For this review, take the finished solid that the model builds, in its own axes (mm). A direction names the side the tool comes from. Round coordinates to 2 decimals unless told otherwise and drop trailing zeros. Write each loop counter-clockwise with the first axis right and the second up, starting at its lowest first coordinate (ties: lowest second). Pieces come first, ordered by that corner, then holes. Notation, with made-up numbers: M 39,9.5 L 82,9.5 A14 ccw 82,22.5 Z; hole C -14,-6.75 d10. An arc over 180 degrees is marked long. Use one line per item in the form item = value. Start each with the question number.
Item 1: Add section B-B (z = 16). State the section outline as (x, y) points (3 decimals).
Item 2: For P1, Ø5, axis at y = 4.5, z = 2, coming from the +X side; P2, Ø2.5, axis at y = 10.91, z = 29.1, coming from the +X side; P3, Ø11.5, axis at y = 20, z = 20, coming from the -X side; P4, Ø3, axis at x = 6.5, z = 16, coming from the +Y side, all flat-tipped, find the tip position at first contact; note any pin that passes through.
Item 3: For line 1 (Z direction, x = 2.5, y = 36.83) (1 decimal); line 2 (Z direction, x = 6, y = 36.5); line 3 (X direction, y = 4, z = 7), list the stretches that pass through material, from the lowest coordinate up. Write a range as [from, to].
Item 4: Add section A-A (y = 19). State the section outline as (x, z) points (3 decimals).
Item 5: Draft analysis for pull direction Y (two halves, no side actions). For faces 1 (the cylindrical face through (3.256, 3.128, 4.253)), 2 (the cylindrical face through (1.25, 28.09, 11.04)), 3 (the flat face through (1, 40.005, 12)), 4 (the flat face through (1, 20, 0)), state which applies: released by +Y, released by -Y, zero draft, split by the parting line, or undercut.
Item 6: Add section C-C (x = 3.25). Count the separate pieces of the cut face and the enclosed holes in it, and give its area (3 significant figures).
Item 7: For faces 5 (the flat face through (1, 40.005, 36)), 6 (the flat face through (6.985, 20, 30)), 7 (the cylindrical face through (6.484, 16.855, 10.009)), list the 3-axis set-ups (+Z, -Z, +X, -X, +Y, -Y) from which the entire face can be reached by the end or side of a thin tool; tool diameter is ignored.
Item 8: Add section D-D (z = 11). State the section outline as (x, y) points (3 decimals).
Autodesk Inventor part; units mm, degrees
ref_plane "YZ Plane" through (0, 0, 0) normal (1, 0, 0) x (0, 1, 0)
ref_plane "XZ Plane" through (0, 0, 0) normal (0, 1, 0) x (-1, 0, 0)
ref_plane "XY Plane" through (0, 0, 0) normal (0, 0, 1) x (1, 0, 0)
sketch "Sketch1" plane through (0, 0, 0) normal (1, 0, 0) x (0, 1, 0)
  line L0 (0, 0) -> (40.005, 0)
  line L1 (40.005, 0) -> (40.005, 40.005)
  line L2 (40.005, 40.005) -> (0, 40.005)
  line L3 (0, 40.005) -> (0, 0)
  dimension "d0" = 40.005
  dimension "d1" = 40.005
extrude "Extrusion1" add sketch "Sketch1" along normal blind 2.54
fillet "Fillet1" radius 3.175 4 edges at (1.27, 40.005, 40.005) (1.27, 0, 40.005) (1.27, 0, 0) (1.27, 40.005, 0)
sketch "Sketch2" plane through (2.54, 0, 0) normal (1, 0, 0) x (0, 0, -1)
  arc A0 (0, 36.83) -> (-3.175, 40.005) centre (-3.175, 36.83) ccw
  arc A1 (-36.83, 40.005) -> (-40.005, 36.83) centre (-36.83, 36.83) ccw
  arc A2 (-40.005, 3.175) -> (-36.83, 0) centre (-36.83, 3.175) ccw
  arc A3 (-3.175, 0) -> (0, 3.175) centre (-3.175, 3.175) ccw
  circle A4 centre (-36.83, 3.175) radius 3.175
  circle A5 centre (-36.83, 36.83) radius 3.175
  circle A6 centre (-3.175, 36.83) radius 3.175
  circle A7 centre (-3.175, 3.175) radius 3.175
  point P0 (0, 0)
extrude "Extrusion2" add sketch "Sketch2" along normal blind 4.064
sketch "Sketch3" plane through (6.604, 3.175, 36.83) normal (1, 0, 0) x (0, 0, -1)
  circle A0 centre (0, 0) radius 3.175
  circle A1 centre (0, 33.655) radius 3.175
  circle A2 centre (33.655, 33.655) radius 3.175
  circle A3 centre (33.655, 0) radius 3.175
  point P0 (36.83, -3.175)
hole "Hole1" at (6.604, 36.83, 36.83) at (6.604, 36.83, 3.175) at (6.604, 3.175, 3.175) at (6.604, 3.175, 36.83) direction (-1, 0, 0) diameter 2.159 end through all
sketch "Sketch4" plane through (2.54, 0, 0) normal (1, 0, 0) x (0, 0, -1)
  arc A0 (-3.175, 40.005) -> (0, 36.83) centre (-3.175, 36.83) ccw
  arc A1 (-36.83, 0) -> (-40.005, 3.175) centre (-36.83, 3.175) ccw
  line L0 (-10.9093, 10.9093) -> (-29.0957, 10.9093)
  line L1 (-29.0957, 10.9093) -> (-29.0957, 29.0957)
  line L2 (-29.0957, 29.0957) -> (-10.9093, 29.0957)
  line L3 (-10.9093, 29.0957) -> (-10.9093, 10.9093)
  line L4 (-36.83, 3.175) -> (-3.175, 36.83) construction
  line L5 (-10.9093, 10.9093) -> (-29.0957, 29.0957) construction
  point P0 (0, 0)
  point P1 (-20.0025, 20.0025)
  dimension "d14" = 18.1864
hole "Hole2" at (2.54, 10.9093, 29.0957) at (2.54, 29.0957, 29.0957) at (2.54, 10.9093, 10.9093) at (2.54, 29.0957, 10.9093) direction (-1, 0, 0) diameter 2.032 end through all
sketch "Sketch5" plane through (2.54, 0, 0) normal (1, 0, 0) x (0, 0, -1)
  circle A0 centre (-10.9093, 10.9093) radius 1.016
  circle A1 centre (-29.0957, 29.0957) radius 1.016
  line L0 (-29.0957, 29.0957) -> (-10.9093, 10.9093) construction
  circle A2 centre (-20.0025, 20.0025) radius 10.4775
  point P0 (0, 0)
  dimension "d23" = 20.955
extrude "Extrusion3" add sketch "Sketch5" along normal blind 8.001 contours A2
sketch "Sketch6" plane through (10.541, 20.0025, 20.0025) normal (1, 0, 0) x (0, 0, -1)
  circle A0 centre (0, 0) radius 10.4775
  circle A1 centre (0, 0) radius 6.35
  point P0 (20.0025, -20.0025)
  dimension "d27" = 6.35
extrude "Extrusion4" cut sketch "Sketch6" against normal through all contours A1
sketch "Sketch7" plane through (10.541, 20.0025, 20.0025) normal (1, 0, 0) x (0, 0, -1)
  circle A0 centre (0, 0) radius 10.4775
  line L0 (-10.4775, -5.4418) -> (-8.9535, -5.4418)
  line L1 (-8.9535, -5.4418) -> (-8.9535, 5.4418)
  line L2 (-8.9535, 5.4418) -> (-10.4775, 5.4418)
  line L3 (-10.4775, 5.4418) -> (-10.4775, -5.4418)
  point P0 (20.0025, -20.0025)
  dimension "d30" = 19.431
extrude "Extrusion5" cut sketch "Sketch7" against normal blind 3.556 contours L1 A0 | A0 L3 L2 | L0 L3 A0 picked at (-9.2326, 1.2437)
sketch "Sketch10" plane through (0, 0, 0) normal (-1, 0, 0) x (0, 0, 1)
  line L0 (3.175, 40.005) -> (36.83, 40.005)
  line L1 (21.5392, 40.005) -> (29.7434, 47.752)
  line L2 (29.7434, 47.752) -> (34.6202, 40.005)
  line L3 (36.83, 0) -> (3.175, 0)
  line L4 (40.005, 36.83) -> (40.005, 3.175)
  point P0 (0, 0)
  dimension "d43" = 5.3848
  dimension "d44" = 10.2616
  dimension "d45" = 18.4658
  dimension "d46" = 47.752
extrude "Extrusion8" add sketch "Sketch10" against normal up to surface (2.54 mm away)
equation "\"d1\" = d0"
properties part number "Face Plate" material "PC/ABS Plastic"
Calculated:
q1.outline = M 0,0 L 2.54,0 L 2.54,10.32 L 10.541,10.32 L 10.541,15.073 L 0,15.073 Z; M 0,24.932 L 10.541,24.932 L 10.541,29.685 L 2.54,29.685 L 2.54,40.005 L 0,40.005 Z
q2.P1 = 6.6
q2.P2 = 2.54
q2.P3 = through
q2.P4 = 30.18
q3.line_1 = [0, 2.1], [4.3, 35.8], [37.9, 40]
q3.line_2 = [0.02, 2.15], [4.2, 6.33], [33.67, 35.8], [37.86, 39.99]
q3.line_3 = [0, 2.54]
q4.outline = M 0,0 L 2.54,0 L 2.54,9.573 L 10.541,9.573 L 10.541,13.732 L 0,13.732 Z; M 0,26.273 L 10.541,26.273 L 10.541,28.956 L 6.985,28.956 L 6.985,30.432 L 2.54,30.432 L 2.54,40.005 L 0,40.005 Z
q5.face_1 = undercut
q5.face_2 = undercut
q5.face_3 = released by +Y
q5.face_4 = zero draft
q6.separate_pieces = 5
q6.enclosed_holes = 5
q6.area = 330 mm^2
q7.face_5 = +Z, +X, -X, +Y
q7.face_6 = +Z, +X, +Y, -Y
q7.face_7 = +X
q8.outline = M 0,0 L 2.54,0 L 2.54,9.897 L 0,9.897 Z; M 0,11.921 L 2.54,11.921 L 2.54,14.642 L 10.541,14.642 L 10.541,25.363 L 2.54,25.363 L 2.54,28.084 L 0,28.084 Z; M 0,30.108 L 2.54,30.108 L 2.54,40.005 L 0,40.005 Z
